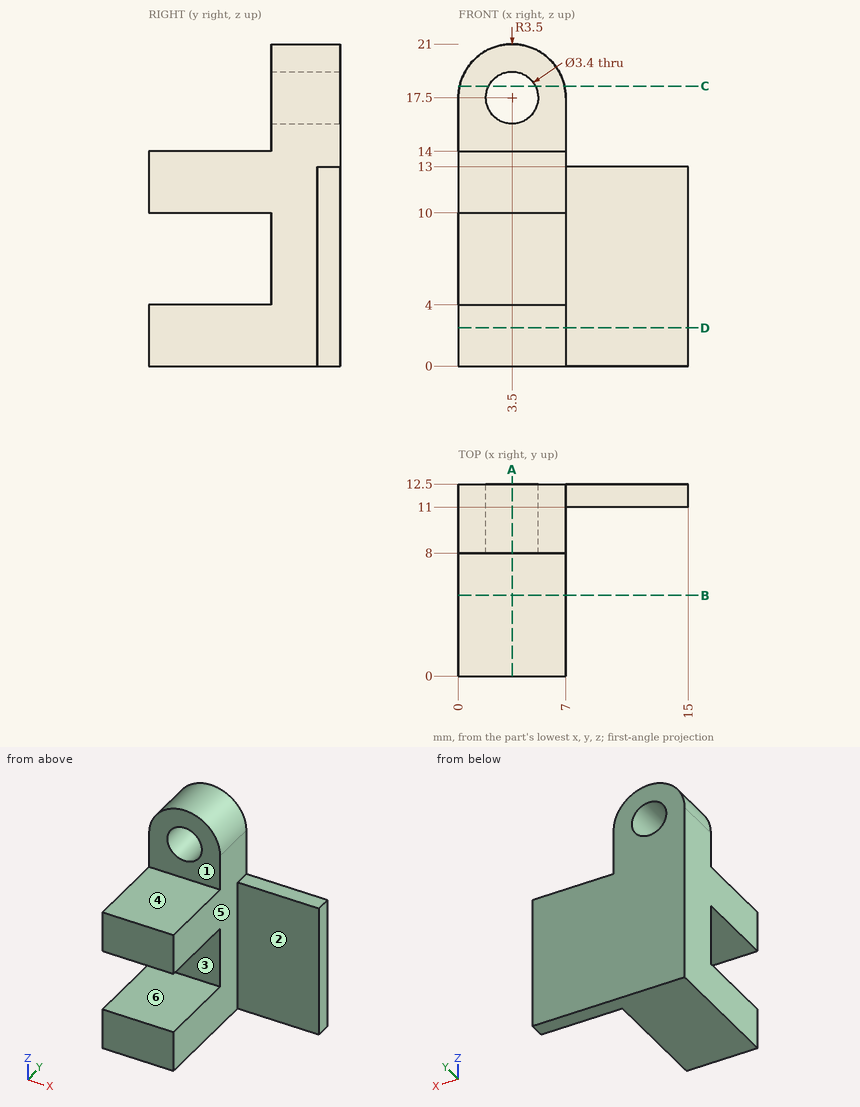
Study the drawing (mm; zero at the part's minimum x, y, z) and answer. A direction names the side the tool comes from. Round coordinates to 2 decimals unless told otherwise and drop trailing zeros. Loops run counter-clockwise (first coordinate to the right, second up) from the corner with the lowest first, then second, coordinate; pieces in that order, holes last. Notation, with made-up numbers: (27.25, -11) -> (56.25, -11) arc R24 cw to (56.25, 28) -> close; hole circle Ø7 at (-16.5, 7). An arc over 180 degrees is marked (long way). One line per item, written item: value.
1) A cutting plane is placed at A-A (x = 3.5). Determine the outline of the cut face in (y, z).
Answer list:
outline: (0, 0) -> (12.5, 0) -> (12.5, 15.8) -> (8, 15.8) -> (8, 14) -> (0, 14) -> (0, 10) -> (8, 10) -> (8, 4) -> (0, 4) -> close; (8, 19.2) -> (12.5, 19.2) -> (12.5, 21) -> (8, 21) -> close
2) A cutting plane is placed at C-C (z = 18.25). Determine the outline of the cut face in (x, y).
Answer list:
outline: (0.08, 8) -> (1.97, 8) -> (1.97, 12.5) -> (0.08, 12.5) -> close; (5.03, 8) -> (6.92, 8) -> (6.92, 12.5) -> (5.03, 12.5) -> close
3) For the marked faces 1, 2 and 3, determine the directions among +Z, -Z, +X, -X, +Y, -Y from which every point of the face is accessible in a straight line to the end or side of a thin tool.
Answer list:
face 1: +Z, +X, -X, -Y
face 2: +Z, -Z, +X, -Y
face 3: +X, -X, -Y
4) The mould has two halves that part along Z. Classify the marked faces 4, 5 and 6: pulls with the +Z half, pulls with the -Z half, needs draft (parallel to the pull), parting line crosses it, or undercut.
Answer list:
face 4: pulls with the +Z half
face 5: needs draft
face 6: undercut
5) A cutting plane is placed at D-D (z = 2.5). Determine the outline of the cut face in (x, y).
Answer list:
outline: (0, 0) -> (7, 0) -> (7, 11) -> (15, 11) -> (15, 12.5) -> (0, 12.5) -> close
6) A cutting plane is placed at B-B (y = 5.25). Determine the outline of the cut face in (x, z).
Answer list:
outline: (0, 0) -> (7, 0) -> (7, 4) -> (0, 4) -> close; (0, 10) -> (7, 10) -> (7, 14) -> (0, 14) -> close
7) Flat-ended cylindrical pins translate along their axes: P1, Ø7.5, axis at x = 2, y = 3.5, coming from the +Z side; P2, Ø4, axis at y = 3.5, z = 9, coming from the +X side; P3, Ø7.5, axis at x = 4.5, z = 18.5, coming from the -Y side. Find the tip coordinate at first contact, or state that the pin passes through.
Answer list:
P1: stops at z = 14
P2: stops at x = 7
P3: stops at y = 8
8) Consider L1, parallel to Z at x = 3.5, y = 11.45; L2, parallel to X at y = 11.5, z = 17.5; L3, parallel to Z at x = 6.75, y = 3.25. Determine where each line is inside the solid, lowest interval first. Write a range as [from, to].
Answer list:
L1: z = [0, 15.8], [19.2, 21]
L2: x = [0, 1.8], [5.2, 7]
L3: z = [0, 4], [10, 14]
